Study the drawing (mm; zero at the part's minimum x, y, z) and answer. A direction names the side the tool comes from. Coordinates: 2 decimals unless noted, no trailing zeros. Order: outer loops, then holes, each group sorted by start corner. A loop starts at its lowest first (then second) coordinate and runs counter-clockwise, first axis right, second up.
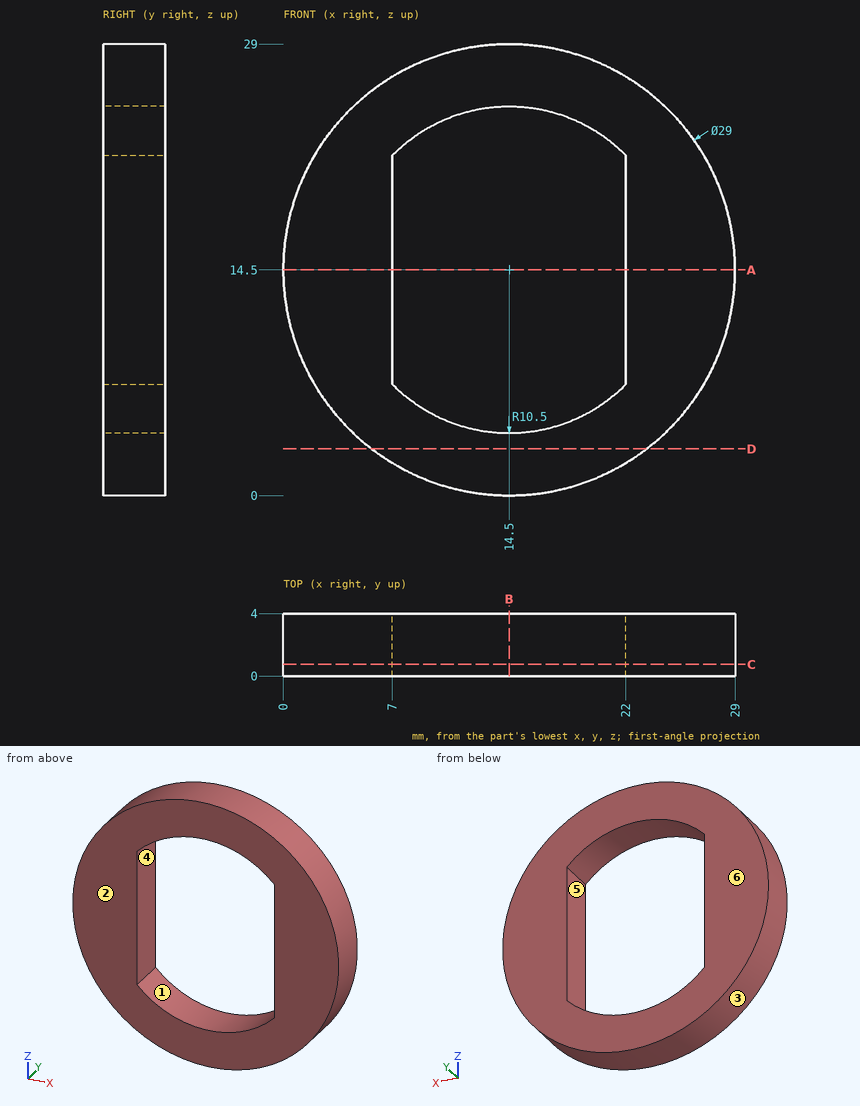
1) Determine the mould class of the marked faces 1, 2, 3 and 4 for opening direction Z: pulls with the +Z half, pulls with the -Z half, needs draft (parallel to the pull), parting line crosses it, or undercut.
A:
face 1: undercut
face 2: needs draft
face 3: parting line crosses it
face 4: undercut
2) A cutting plane is placed at D-D, the plane z = 3. Determine the outline of the cut face in (x, y).
A:
outline: (5.67, 0) - (23.33, 0) - (23.33, 4) - (5.67, 4) - close
3) A cutting plane is placed at B-B, the plane x = 14.5. Determine the outline of the cut face in (y, z).
A:
outline: (0, 0) - (4, 0) - (4, 4) - (0, 4) - close; (0, 25) - (4, 25) - (4, 29) - (0, 29) - close
4) A cutting plane is placed at C-C, the plane y = 0.75. Determine the outline of the cut face in (x, z), and give its area (3 significant figures).
A:
outline: circle Ø29 at (14.5, 14.5); hole (7, 7.15) arc R10.5 ccw to (22, 7.15) - (22, 21.85) arc R10.5 ccw to (7, 21.85) - close
area: 375 mm2
5) Which of the six approach directions +Z, -Z, +X, -X, +Y, -Y give full straight-line access (tool end or side, diameter ignored) to the marked faces 5 and 6?
A:
face 5: +Y, -Y
face 6: +Z, -Z, +X, -X, +Y
6) Straight lines are drawn through the part: line 1 (X direction, y = 2.6, z = 14.75); line 2 (Z direction, x = 14.75, y = 0.7); line 3 (X direction, y = 0.85, z = 10.25). For each, find the intervals that lie inside material, in ascending order.
A:
line 1: x = 0 to 7, 22 to 29
line 2: z = 0 to 4, 25 to 29
line 3: x = 0.64 to 7, 22 to 28.36
7) A cutting plane is placed at A-A, the plane z = 14.5. Determine the outline of the cut face in (x, y), and give its area (3 significant figures).
A:
outline: (0, 0) - (7, 0) - (7, 4) - (0, 4) - close; (22, 0) - (29, 0) - (29, 4) - (22, 4) - close
area: 56.0 mm2
